```python
from build123d import *

# Parameters (mm, degrees)
SKETCH_R     = 5
PAD_DEPTH    = 5
SKETCH002_R  = 26
PAD001_DEPTH = 150
SKETCH001_R  = 21.829625
POCKET_DEPTH = 150


with BuildPart() as part:
    # Sketch → Pad (new body)
    with BuildSketch(Plane.XY):
        with BuildLine():
            Line((-29.76506, -39.750771), (30.181718, -39.750771))
            ThreePointArc((30.181718, -39.750771), (36.954256, -36.945494), (39.759533, -30.172956))
            Line((39.759533, -30.172956), (39.759533, 31.470314))
            ThreePointArc((39.759533, 31.470314), (36.97817, 38.185117), (30.263367, 40.96648))
            Line((30.263367, 40.96648), (-29.735014, 40.96648))
            ThreePointArc((-29.735014, 40.96648), (-36.449803, 38.185124), (-39.231159, 31.470335))
            Line((-39.231159, 31.470335), (-39.231159, -30.284672))
            ThreePointArc((-39.231159, -30.284672), (-36.458603, -36.978215), (-29.76506, -39.750771))
        make_face()
        with Locations((-29.735014, 29.743769)):
            Circle(SKETCH_R, mode=Mode.SUBTRACT)
        with Locations((30.263367, 29.743769)):
            Circle(SKETCH_R, mode=Mode.SUBTRACT)
        with Locations((-29.735014, -30.254622)):
            Circle(SKETCH_R, mode=Mode.SUBTRACT)
        with Locations((30.263367, -30.254622)):
            Circle(SKETCH_R, mode=Mode.SUBTRACT)
    extrude(amount=PAD_DEPTH)

    # Sketch002 → Pad001 (join)
    with BuildSketch(Plane.XY):
        with Locations((0.332326, 0.20453)):
            Circle(SKETCH002_R)
    extrude(amount=PAD001_DEPTH)

    # Sketch001 (on Face13 of Pad) → Pocket (cut)
    with BuildSketch(Plane(origin=(0, 0, 0), x_dir=(1, 0, 0), z_dir=(0, 0, -1))):
        Circle(SKETCH001_R)
    extrude(amount=-POCKET_DEPTH, mode=Mode.SUBTRACT)


solid = part.part
```
Work out the finished part from the listing and answer in its coordinate system (mm). A direction names the side the tool comes from. Give positions to 0.01 mm unless a question says otherwise; leave off trailing zeros. Order: outer loops, then holes, each group sorted by start corner. A loop starts at its lowest first (then second) coordinate and runs counter-clockwise, first axis right, second up.
1. For faces 1 (the flat face through (-18, 19, 5)), 2 (the cylindrical face through (36.9, -37, 2.5)), determine the directions among +Z, -Z, +X, -X, +Y, -Y from which every point of the face is accessible in a straight line to the end or side of a thin tool.
Result sheet:
face 1: +Z
face 2: +Z, -Z, +X, -Y
2. Each of these flat-tipped pins is pushed along its axis until it touches: P1, Ø1, axis at x = -4, z = 126.5, coming from the -Y side; P2, Ø12, axis at x = -29.5, z = 113, coming from the -Y side; P3, Ø23.5, axis at x = 14.5, y = -15.5, coming from the +Z side; P4, Ø2, axis at x = -10.5, z = 39.5, coming from the -Y side. Where does it stop, or does it pass through?
Result sheet:
P1: stops at y = -25.51
P2: stops at y = -10.19
P3: stops at z = 150
P4: stops at y = -23.86
3. Straight lines are drawn through the part: L1, parallel to Y at x = -0.5, z = 96.5; L2, parallel to Z at x = 26, y = 33.5; L3, parallel to Y at x = -2.5, z = 48. For each, find the intervals that lie inside material, in ascending order.
Result sheet:
L1: y = -25.78 to -21.82, 21.82 to 26.19
L2: z = 0 to 5
L3: y = -25.64 to -21.69, 21.69 to 26.05
4. Section A-A, the plane x = -0.5 is taken. Determine the outline of the cut face in (y, z), and give its area (3 significant figures).
Result sheet:
outline: (-39.75, 0) - (-21.82, 0) - (-21.82, 150) - (-25.78, 150) - (-25.78, 5) - (-39.75, 5) - close; (21.82, 0) - (40.97, 0) - (40.97, 5) - (26.19, 5) - (26.19, 150) - (21.82, 150) - close
area: 1,390 mm2
5. Section C-C, the plane z = 44 is taken. Determine the outline of the cut face in (x, y), and give its area (3 significant figures).
Result sheet:
outline: circle Ø52 at (0.33, 0.2); hole circle Ø43.66 at (0, 0)
area: 627 mm2
6. Section B-B, the plane y = 15.5 is taken. Determine the outline of the cut face in (x, z).
Result sheet:
outline: (-39.23, 0) - (-15.37, 0) - (-15.37, 150) - (-20.69, 150) - (-20.69, 5) - (-39.23, 5) - close; (15.37, 0) - (39.76, 0) - (39.76, 5) - (21.36, 5) - (21.36, 150) - (15.37, 150) - close
7. The mould has two halves that part along Y. Classify faces 3 (the flat face through (-39.231, 1, 2)), 4 (the cylindrical face through (26.3, -33.3, 2.5)), 5 (the cylindrical face through (25.132, 8.014, 76.485)): released by +Y, released by -Y, zero draft, split by the parting line, or undercut.
Result sheet:
face 3: zero draft
face 4: undercut
face 5: split by the parting line
